The drawing under review shows one solid part. Ordinate dimensions are in mm from its lowest x, y, z. Give positions to 0.01 mm unless a question says otherwise; leave off trailing zeros. Order: outer loops, then holes, each group sorted by start corner. A loop starts at its lowest first (then second) coordinate and runs counter-clockwise, first axis right, second up. Notation, with made-up numbers: (39, 10) -> (59, 10) arc R20 ccw to (59, 32) -> close; hole circle Ø5 at (36.25, -35.75). An arc over 180 degrees is marked (long way). One line per item, written item: value.
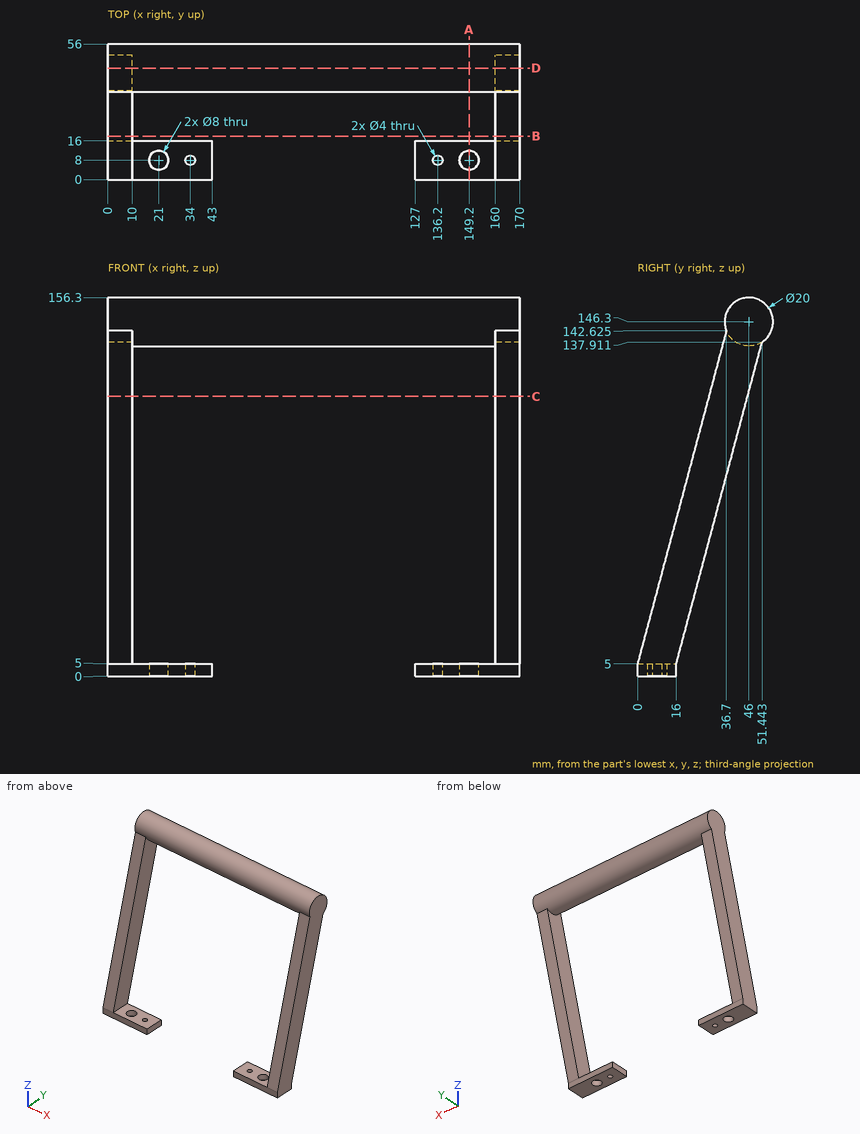
Item 1: Clearance check with flat-ended pins moving along their axes: P1, Ø9, axis at x = 149.2, y = 8, coming from the +Z side; P2, Ø5.5, axis at x = 145.5, z = 3.5, coming from the +Y side; P3, Ø8, axis at x = 147.5, z = 131.5, coming from the +Y side. State where each tip first meets the part, or that it passes through.
Returned:
P1: z = 5
P2: y = 16
P3: through
Item 2: Add section B-B on y = 18. Give the boundary of the cut face in (x, z), plus the area to 3 significant figures.
Returned:
outline: (0, 12.5) -> (10, 12.5) -> (10, 72.5) -> (0, 72.5) -> close; (160, 12.5) -> (170, 12.5) -> (170, 72.5) -> (160, 72.5) -> close
area: 1,200 mm²
Item 3: To check wall thickness, follow line 1 along X through (y, z) = (8, 1.75); line 2 along Y through (x, z) = (34, 1.9); line 3 along X through (y, z) = (22.5, 45). State the ranges of each line that lie inside material, in increasing order. Write a range as from..to.
Returned:
line 1: 0..17, 25..32, 36..43, 127..134.2, 138.2..145.2, 153.2..170
line 2: 0..6, 10..16
line 3: 0..10, 160..170
Item 4: Add section D-D on y = 46. Give the boundary of the cut face in (x, z), plus the area to 3 significant figures.
Returned:
outline: (0, 117.5) -> (10, 117.5) -> (10, 136.3) -> (160, 136.3) -> (160, 117.5) -> (170, 117.5) -> (170, 156.3) -> (0, 156.3) -> close
area: 3,780 mm²
Item 5: Add section A-A on x = 149.2. Give the boundary of the cut face in (y, z), plus the area to 3 significant figures.
Returned:
outline: (0, 0) -> (4, 0) -> (4, 5) -> (0, 5) -> close; (12, 0) -> (16, 0) -> (16, 5) -> (12, 5) -> close; circle Ø20 at (46, 146.3)
area: 354 mm²
Item 6: Add section C-C on z = 115.5. Give the boundary of the cut face in (x, y), plus the area to 3 significant figures.
Returned:
outline: (0, 29.47) -> (10, 29.47) -> (10, 45.47) -> (0, 45.47) -> close; (160, 29.47) -> (170, 29.47) -> (170, 45.47) -> (160, 45.47) -> close
area: 320 mm²
